Check sheet for the modelled part. Datum: model origin and axes. Units: mm. Face numbers are marked on the shaded views. Round coordinates to 2 decimals unless told otherwise and drop trailing zeros. Order: outer loops, then holes, each group sorted by start corner. A loop starts at its lowest first (then second) coordinate and runs counter-clockwise, first axis right, second up.
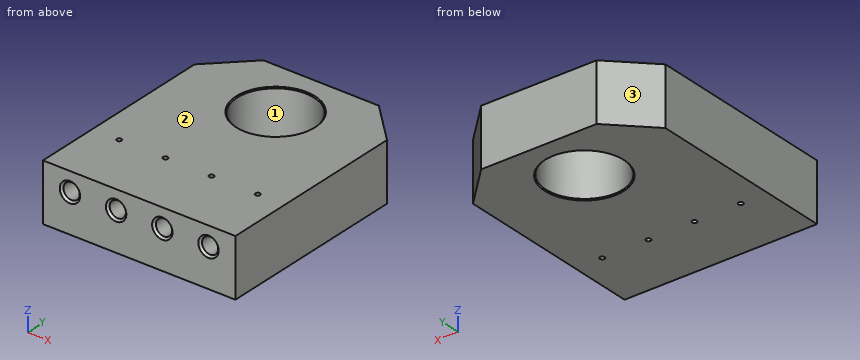
```python
from build123d import *

# Parameters (mm, degrees)
SKETCH1_W                         = 127
SKETCH1_H                         = 152.4
EXTRUDE1_DEPTH                    = 38.1
CHAMFER1_SIZE                     = 25.4
F_1_2_13_TAPPED_HOLE1_D           = 10.71626
F_1_2_13_TAPPED_HOLE1_DEPTH       = 44.45
F_1_2_13_TAPPED_HOLE1_CSINK_D     = 13.462
F_1_2_13_TAPPED_HOLE1_CSINK_ANGLE = 90
F_1_2_13_TAPPED_HOLE1_TIP         = 3.219489309
SKETCH4_R                         = 1.5875
CUT_EXTRUDE1_DEPTH                = 39.1


with BuildPart() as part:
    # Sketch1 → Extrude1 (new body)
    with BuildSketch(Plane.XY):
        with Locations((63.5, 76.2)):
            Rectangle(SKETCH1_W, SKETCH1_H)
    extrude(amount=EXTRUDE1_DEPTH)

    # Sketch5 → 1 (1) Diameter Hole1 (revolve, cut)
    with BuildSketch(Plane(origin=(63.5, 114.3, 38.1), x_dir=(0, -1, 0), z_dir=(1, 0, 0))):
        Polygon((0, 0), (0, 38.1), (26.0985, 38.1), (25.4635, 37.465), (25.4635, 0.635), (26.0985, 0), align=None)
    revolve(axis=Axis((63.5, 114.3, 44.45), (0, 0, -1)), mode=Mode.SUBTRACT)

    # Chamfer1
    chamfer1_edges = [part.edges().sort_by_distance(p)[0] for p in [
        (0, 152.4, 19.05),
        (127, 152.4, 19.05),
    ]]
    chamfer(chamfer1_edges, length=CHAMFER1_SIZE)

    # 1/2-13 Tapped Hole1
    with Locations(Plane(origin=(109.22, 0, 25.4), x_dir=(0, 0, -1), z_dir=(0, -1, 0))):
        with Locations((0, 0), (0, -30.48), (0, -60.96), (0, -91.44)):
            CounterSinkHole(F_1_2_13_TAPPED_HOLE1_D / 2, F_1_2_13_TAPPED_HOLE1_CSINK_D / 2, depth=F_1_2_13_TAPPED_HOLE1_DEPTH, counter_sink_angle=F_1_2_13_TAPPED_HOLE1_CSINK_ANGLE)
            with Locations((0, 0, -(F_1_2_13_TAPPED_HOLE1_DEPTH + F_1_2_13_TAPPED_HOLE1_TIP / 2))):  # 118° drill point
                Cone(0, F_1_2_13_TAPPED_HOLE1_D / 2, F_1_2_13_TAPPED_HOLE1_TIP, mode=Mode.SUBTRACT)

    # Sketch4 → Cut-Extrude1 (cut, through all)
    with BuildSketch(Plane.XY.offset(38.1)):
        with Locations((17.78, 41.275)):
            Circle(SKETCH4_R)
        with Locations((48.26, 41.275)):
            Circle(SKETCH4_R)
        with Locations((78.74, 41.275)):
            Circle(SKETCH4_R)
        with Locations((109.22, 41.275)):
            Circle(SKETCH4_R)
    extrude(amount=-CUT_EXTRUDE1_DEPTH, mode=Mode.SUBTRACT)


solid = part.part
```
Item 1: Scan lines: line 1 along X through (y, z) = (35, 25.4); line 2 along X through (y, z) = (114.5, 6); line 3 along Y through (x, z) = (78, 32). Record each from-to range of solid material in increasing order.
Answer:
line 1: x = 0 to 12.42, 23.14 to 42.9, 53.62 to 73.38, 84.1 to 103.86, 114.58 to 127
line 2: x = 0 to 38.04, 88.96 to 127
line 3: y = 0.09 to 39.87, 42.68 to 93.37, 135.23 to 152.4
Item 2: Go/stop test with flat-tipped pins: P1, Ø12.5, axis at x = 109.22, z = 25.4, coming from the -Y side; P2, Ø1.5, axis at y = 134.5, z = 12.5, coming from the +X side; P3, Ø9.5, axis at x = 48.26, z = 25.4, coming from the -Y side. Record where each tip stops, or that it passes through.
Answer:
P1: stops at y = 0.48
P2: stops at x = 120.25
P3: stops at y = 44.82
Item 3: Sectioned sample at A-A (y = 36). Record the cut outline in (x, z).
Answer:
outline: (0, 0) - (127, 0) - (127, 38.1) - (0, 38.1) - close; hole circle Ø10.72 at (17.78, 25.4); hole circle Ø10.72 at (48.26, 25.4); hole circle Ø10.72 at (78.74, 25.4); hole circle Ø10.72 at (109.22, 25.4)
Item 4: Sectioned sample at B-B (x = 63.5). Record the cut outline in (y, z) (1 decimal), and give its area (3 significant figures).
Answer:
outline: (0, 0) - (88.2, 0) - (88.8, 0.6) - (88.8, 37.5) - (88.2, 38.1) - (0, 38.1) - close; (139.8, 0.6) - (140.4, 0) - (152.4, 0) - (152.4, 38.1) - (140.4, 38.1) - (139.8, 37.5) - close
area: 3,870 mm2
Item 5: Release check for a two-part mould opening along Y. For the marked faces 1, 2 and 3 record: released by +Y, released by -Y, zero draft, split by the parting line, or undercut.
Answer:
face 1: undercut
face 2: zero draft
face 3: released by +Y
Item 6: Sectioned sample at C-C (z = 6). Record the cut outline in (x, y) (1 decimal).
Answer:
outline: (0, 0) - (127, 0) - (127, 127) - (101.6, 152.4) - (25.4, 152.4) - (0, 127) - close; hole circle Ø3.2 at (17.8, 41.3); hole circle Ø50.9 at (63.5, 114.3); hole circle Ø3.2 at (48.3, 41.3); hole circle Ø3.2 at (78.7, 41.3); hole circle Ø3.2 at (109.2, 41.3)
